CAD build for the part. Positions are in the model's coordinates, mm. A direction names the side the tool comes from. Give positions to 0.01 mm unless a question says otherwise; leave off trailing zeros. Write each loop counter-clockwise with the first axis right and the second up, starting at its lowest first coordinate (ties: lowest second). Pieces come first, ordered by that corner, then holes. Notation, with made-up numbers: (51.25, -8.75) -> (64.25, -8.75) arc R6 cw to (64.25, -0.75) -> close; hole circle Ø2 at (89, 35.25). An arc over 180 degrees is marked (long way). Answer as a JSON object with one key per item and string values.
```python
from build123d import *

# Parameters (mm, degrees)
F1_DEPTH = 4
F2_W     = 300
F2_H     = 7
F3_DEPTH = 1.5
F4_DEPTH = 2.5


with BuildPart() as f1:
    # F0 (on Top) → F1 (new body)
    with BuildSketch(Plane.XY):
        with BuildLine():
            Line((-4.287656, -89.914214), (295.712344, -89.914214))
            Line((295.712344, -89.914214), (295.712344, 79.085786))
            ThreePointArc((295.712344, 79.085786), (295.41945, 79.792893), (294.712344, 80.085786))
            Line((294.712344, 80.085786), (-3.287656, 80.085786))
            ThreePointArc((-3.287656, 80.085786), (-3.994763, 79.792893), (-4.287656, 79.085786))
            Line((-4.287656, 79.085786), (-4.287656, -89.914214))
        make_face()
        with BuildLine():
            ThreePointArc((180.696579, 55.444697), (183.525006, 56.61627), (186.353433, 55.444697))
            Line((186.353433, 55.444697), (291.712344, -49.914214))
            Line((291.712344, -49.914214), (289.23747, -52.389087))
            Line((289.23747, -52.389087), (184.232113, 52.61627))
            ThreePointArc((184.232113, 52.61627), (183.525006, 52.909163), (182.817899, 52.61627))
            Line((182.817899, 52.61627), (160.897589, 30.695959))
            ThreePointArc((160.897589, 30.695959), (160.604696, 29.988853), (160.897589, 29.281746))
            Line((160.897589, 29.281746), (236.911568, -46.732233))
            ThreePointArc((236.911568, -46.732233), (237.618675, -47.025126), (238.325782, -46.732233))
            Line((238.325782, -46.732233), (238.679335, -46.37868))
            Line((238.679335, -46.37868), (266.963606, -74.662951))
            Line((266.963606, -74.662951), (265.902946, -75.723611))
            Line((265.902946, -75.723611), (263.428072, -78.198485))
            Line((263.428072, -78.198485), (155.240735, 29.988853))
            Line((155.240735, 29.988853), (132.259764, 52.969823))
            ThreePointArc((132.259764, 52.969823), (131.552658, 53.262716), (130.845551, 52.969823))
            Line((130.845551, 52.969823), (108.925241, 31.049513))
            ThreePointArc((108.925241, 31.049513), (108.632347, 30.342406), (108.925241, 29.635299))
            Line((108.925241, 29.635299), (184.93922, -46.37868))
            ThreePointArc((184.93922, -46.37868), (185.646326, -46.671573), (186.353433, -46.37868))
            Line((186.353433, -46.37868), (186.706987, -46.025126))
            Line((186.706987, -46.025126), (214.991258, -74.309398))
            Line((214.991258, -74.309398), (213.930598, -75.370058))
            Line((213.930598, -75.370058), (211.455724, -77.844931))
            Line((211.455724, -77.844931), (103.268386, 30.342406))
            Line((103.268386, 30.342406), (80.287416, 53.323376))
            ThreePointArc((80.287416, 53.323376), (79.580309, 53.61627), (78.873202, 53.323376))
            Line((78.873202, 53.323376), (56.952892, 31.403066))
            ThreePointArc((56.952892, 31.403066), (56.659999, 30.695959), (56.952892, 29.988853))
            Line((56.952892, 29.988853), (132.966871, -46.025126))
            ThreePointArc((132.966871, -46.025126), (133.673978, -46.318019), (134.381085, -46.025126))
            Line((134.381085, -46.025126), (134.734638, -45.671573))
            Line((134.734638, -45.671573), (163.018909, -73.955844))
            Line((163.018909, -73.955844), (161.958249, -75.016504))
            Line((161.958249, -75.016504), (159.483376, -77.491378))
            Line((159.483376, -77.491378), (51.296038, 30.695959))
            Line((51.296038, 30.695959), (28.315068, 53.67693))
            ThreePointArc((28.315068, 53.67693), (27.607961, 53.969823), (26.900854, 53.67693))
            Line((26.900854, 53.67693), (4.980544, 31.75662))
            ThreePointArc((4.980544, 31.75662), (4.687651, 31.049513), (4.980544, 30.342406))
            Line((4.980544, 30.342406), (52.710252, -17.387302))
            ThreePointArc((52.710252, -17.387302), (53.417358, -17.680195), (54.124465, -17.387302))
            Line((54.124465, -17.387302), (54.478019, -17.033748))
            Line((54.478019, -17.033748), (111.046561, -73.602291))
            Line((111.046561, -73.602291), (109.985901, -74.662951))
            Line((109.985901, -74.662951), (107.511027, -77.137825))
            Line((107.511027, -77.137825), (-0.67631, 31.049513))
            Line((-0.67631, 31.049513), (24.779534, 56.505357))
            ThreePointArc((24.779534, 56.505357), (27.607961, 57.67693), (30.436388, 56.505357))
            Line((30.436388, 56.505357), (53.770912, 33.170833))
            Line((53.770912, 33.170833), (76.751882, 56.151804))
            ThreePointArc((76.751882, 56.151804), (79.580309, 57.323376), (82.408736, 56.151804))
            Line((82.408736, 56.151804), (105.74326, 32.81728))
            Line((105.74326, 32.81728), (128.724231, 55.79825))
            ThreePointArc((128.724231, 55.79825), (131.552658, 56.969823), (134.381085, 55.79825))
            Line((134.381085, 55.79825), (157.715609, 32.463726))
            Line((157.715609, 32.463726), (180.696579, 55.444697))
        make_face(mode=Mode.SUBTRACT)
    extrude(amount=F1_DEPTH)

    # F2 (on face) → F3 (cut)
    with BuildSketch(Plane(origin=(0, 0, 0), x_dir=(1, 0, 0), z_dir=(0, 0, -1))):
        with Locations((145.712344, 86.414214)):
            Rectangle(F2_W, F2_H)
    extrude(amount=-F3_DEPTH, mode=Mode.SUBTRACT)

    # F2 (on face) → F4 (cut)
    with BuildSketch(Plane(origin=(0, 0, 0), x_dir=(1, 0, 0), z_dir=(0, 0, -1))):
        Polygon((118.117629, 66.531223), (111.046561, 73.602291), (54.478019, 17.033748), (61.549086, 9.96268), align=None)
        Polygon((170.089977, 66.884776), (163.018909, 73.955844), (134.734638, 45.671573), (141.805706, 38.600505), align=None)
        Polygon((222.062326, 67.23833), (214.991258, 74.309398), (186.706987, 46.025126), (193.778054, 38.954058), align=None)
        Polygon((274.034674, 67.591883), (266.963606, 74.662951), (238.679335, 46.37868), (245.750403, 39.307612), align=None)
    extrude(amount=-F4_DEPTH, mode=Mode.SUBTRACT)


solid = f1.part
```
1) Slice it at D-D (x = 203). List the corners of the cut face in (y, z), then the cut area to 3 significant figures.
Model answer:
{"outline": "(-89.91, 1.5) -> (-82.91, 1.5) -> (-82.91, 0) -> (-69.39, 0) -> (-69.39, 4) -> (-89.91, 4) -> close; (-62.32, 2.5) -> (-48.18, 2.5) -> (-48.18, 0) -> (-17.77, 0) -> (-17.77, 4) -> (-62.32, 4) -> close; (-12.82, 0) -> (33.85, 0) -> (33.85, 4) -> (-12.82, 4) -> close; (38.8, 0) -> (80.09, 0) -> (80.09, 4) -> (38.8, 4) -> close", "area": "566 mm2"}
2) Wall check: probe 1 along Y at (x, z) = (29.5, 0.55); probe 2 along Y at (x, z) = (215.5, 0.3); probe 3 along X at (y, z) = (17.5, 0.6). Give the ranges that are in metal, low to high.
Model answer:
{"probe 1": "y = -82.91 to 0.87, 5.82 to 52.49, 57.2 to 80.09", "probe 2": "y = -82.91 to -73.8, -60.68 to -30.27, -25.32 to 21.35, 26.3 to 80.09", "probe 3": "x = -4.29 to 12.87, 17.82 to 64.49, 69.44 to 116.11, 121.06 to 167.73, 172.68 to 219.35, 224.3 to 295.71"}
3) Slice it at C-C (y = 17.5). List the corners of the cut face in (x, z).
Model answer:
{"outline": "(-4.29, 0) -> (12.87, 0) -> (12.87, 4) -> (-4.29, 4) -> close; (17.82, 0) -> (64.49, 0) -> (64.49, 4) -> (17.82, 4) -> close; (69.44, 0) -> (116.11, 0) -> (116.11, 4) -> (69.44, 4) -> close; (121.06, 0) -> (167.73, 0) -> (167.73, 4) -> (121.06, 4) -> close; (172.68, 0) -> (219.35, 0) -> (219.35, 4) -> (172.68, 4) -> close; (224.3, 0) -> (295.71, 0) -> (295.71, 4) -> (224.3, 4) -> close"}
4) 3-axis set-ups, long thin cutter, end or side, ignore diameter. For faces 3 (the flat face through (144, -86, 1.5)), 4 (the flat face through (94.43, -7.49, 1.97)), 5 (the flat face through (241.99, -43.07, 1.08)): which of +Z, -Z, +X, -X, +Y, -Y reach the whole face in a straight line?
Model answer:
{"face 3": "-Z, +X, -X, -Y", "face 4": "+Z, -Z", "face 5": "-Z"}
5) Slice it at A-A (y = -58). List the corners of the cut face in (x, z).
Model answer:
{"outline": "(-4.29, 0) -> (88.37, 0) -> (88.37, 4) -> (-4.29, 4) -> close; (95.44, 2.5) -> (109.59, 2.5) -> (109.59, 0) -> (139.99, 0) -> (139.99, 4) -> (95.44, 4) -> close; (147.06, 2.5) -> (161.21, 2.5) -> (161.21, 0) -> (191.61, 0) -> (191.61, 4) -> (147.06, 4) -> close; (198.68, 2.5) -> (212.82, 2.5) -> (212.82, 0) -> (243.23, 0) -> (243.23, 4) -> (198.68, 4) -> close; (250.3, 2.5) -> (264.44, 2.5) -> (264.44, 0) -> (295.71, 0) -> (295.71, 4) -> (250.3, 4) -> close"}
6) Mould opens along X. For faces 1 (the flat face through (252.6, -60.3, 3.2)), 2 (the flat face through (144, -4, 4)) say: released by +X, released by -X, zero draft, split by the parting line, or undercut.
Model answer:
{"face 1": "undercut", "face 2": "zero draft"}
7) Slice it at B-B (x = 46). List the corners of the cut face in (y, z).
Model answer:
{"outline": "(-89.91, 1.5) -> (-82.91, 1.5) -> (-82.91, 0) -> (-15.63, 0) -> (-15.63, 4) -> (-89.91, 4) -> close; (-10.68, 0) -> (35.99, 0) -> (35.99, 4) -> (-10.68, 4) -> close; (40.94, 0) -> (80.09, 0) -> (80.09, 4) -> (40.94, 4) -> close"}
